```python
from build123d import *

# Parameters (mm, degrees)
F0_R      = 2.95
F1_DEPTH  = 4
F2_W      = 8.5
F2_H      = 8.5
F3_DEPTH  = 1
F4_R      = 1.5
F5_DEPTH  = 3
F7_DEPTH  = 4
F8_R      = 1.5
F9_DEPTH  = 3
F10_W     = 48
F10_H     = 4
F11_DEPTH = 1
F12_W     = 40
F12_H     = 1
F13_DEPTH = 3
F14_W     = 7
F14_H     = 7
F14_R     = 2.95
F15_DEPTH = 2


# Not quite as in the source:
# - a feature names something its author has since deleted; it is built from what else it names


with BuildPart() as f1:
    # F0 (on Top) → F1 (new body)
    with BuildSketch(Plane.XY):
        Polygon((-24, -33), (24, -33), (24, 26.5), (24, 35), (17.5, 35), (-17.5, 35), (-24, 35), (-24, 26.5), align=None)
        Circle(F0_R, mode=Mode.SUBTRACT)
    extrude(amount=F1_DEPTH)

    # F2 (on face) → F3 (cut)
    with BuildSketch(Plane(origin=(0, 0, 0), x_dir=(1, 0, 0), z_dir=(0, 0, -1))):
        with Locations((19.75, -30.75)):
            Rectangle(F2_W, F2_H)
        with Locations((-19.75, -30.75)):
            Rectangle(F2_W, F2_H)
    extrude(amount=-F3_DEPTH, mode=Mode.SUBTRACT)

    # F4 (on face) → F5 (cut)
    with BuildSketch(Plane(origin=(0, 0, 1), x_dir=(1, 0, 0), z_dir=(0, 0, -1))):
        with Locations((18.7980970389, -29.7980970389)):
            Circle(F4_R)
    extrude(amount=-F5_DEPTH, mode=Mode.SUBTRACT)

    # F6 (on face) → F7 (cut)
    with BuildSketch(Plane.XY.offset(4)):
        with BuildLine():
            Line((-18.7027541446, 3), (-11.1018016556, 3))
            ThreePointArc((-11.1018016556, 3), (-8.1134067433, 8.1500080379), (-2.95, 11.115192306))
            Line((-2.95, 11.115192306), (-2.95, 23.25))
            Line((-2.95, 23.25), (-18.7027541446, 23.25))
            Line((-18.7027541446, 23.25), (-18.7027541446, 3))
        make_face()
        with BuildLine():
            Line((2.95, 23.25), (2.95, 11.115192306))
            ThreePointArc((2.95, 11.115192306), (8.1134067433, 8.1500080379), (11.1018016556, 3))
            Line((11.1018016556, 3), (18.7027541446, 3))
            Line((18.7027541446, 3), (18.7027541446, 23.25))
            Line((18.7027541446, 23.25), (2.95, 23.25))
        make_face()
        with BuildLine():
            Line((-18.7027541446, -9.125), (-18.7027541446, -16.125))
            Line((-18.7027541446, -16.125), (-18.7027541446, -26.1487078986))
            Line((-18.7027541446, -26.1487078986), (-10, -26.1487078986))
            Line((-10, -26.1487078986), (-2.95, -26.1487078986))
            Line((-2.95, -26.1487078986), (-2.95, -11.115192306))
            ThreePointArc((-2.95, -11.115192306), (-8.1134067433, -8.1500080379), (-11.1018016556, -3))
            Line((-11.1018016556, -3), (-17.7254807204, -3))
            Line((-17.7254807204, -3), (-18.7027541446, -3))
            Line((-18.7027541446, -3), (-18.7027541446, -9.125))
        make_face()
        with BuildLine():
            ThreePointArc((11.1018016556, -3), (8.1134067433, -8.1500080379), (2.95, -11.115192306))
            Line((2.95, -11.115192306), (2.95, -26.1487078986))
            Line((2.95, -26.1487078986), (10, -26.1487078986))
            Line((10, -26.1487078986), (18.7027541446, -26.1487078986))
            Line((18.7027541446, -26.1487078986), (18.7027541446, -16.125))
            Line((18.7027541446, -16.125), (18.7027541446, -9.125))
            Line((18.7027541446, -9.125), (18.7027541446, -3.9093415253))
            Line((18.7027541446, -3.9093415253), (18.7027541446, -3))
            Line((18.7027541446, -3), (11.1018016556, -3))
        make_face()
    extrude(amount=-F7_DEPTH, mode=Mode.SUBTRACT)

    # F8 (on face) → F9 (cut)
    with BuildSketch(Plane(origin=(0, 0, 1), x_dir=(1, 0, 0), z_dir=(0, 0, -1))):
        with Locations((-18.7980970389, -29.7980970389)):
            Circle(F8_R)
    extrude(amount=-F9_DEPTH, mode=Mode.SUBTRACT)

    # F10 (on face) → F11 (cut)
    with BuildSketch(Plane(origin=(0, 0, 0), x_dir=(1, 0, 0), z_dir=(0, 0, -1))):
        with Locations((0, 31)):
            Rectangle(F10_W, F10_H)
    extrude(amount=-F11_DEPTH, mode=Mode.SUBTRACT)

    # F12 (on face) → F13 (cut)
    with BuildSketch(Plane(origin=(0, 0, 1), x_dir=(1, 0, 0), z_dir=(0, 0, -1))):
        with Locations((0, 31)):
            Rectangle(F12_W, F12_H)
    extrude(amount=-F13_DEPTH, mode=Mode.SUBTRACT)

    # F14 (on face) → F15 (cut)
    with BuildSketch(Plane.XY.offset(4)):
        Rectangle(F14_W, F14_H)
        Circle(F14_R, mode=Mode.SUBTRACT)
    extrude(amount=-F15_DEPTH, mode=Mode.SUBTRACT)


solid = f1.part
```
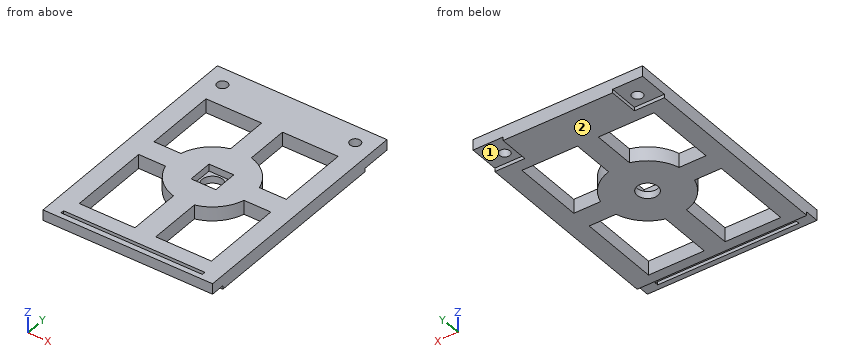
For this review, take the finished solid that the model builds, in its own axes (mm). Face numbers are marked on the shaded views. A direction names the side the tool comes from. Coordinates: 2 decimals unless noted, no trailing zeros. Loops run counter-clockwise (first coordinate to the right, second up) from the corner with the lowest first, then second, coordinate; pieces in that order, holes last.
1. Add section D-D, the plane x = 7. Give the boundary of the cut face in (y, z).
2. For line 1 (X direction, y = 18, z = 3); line 2 (Y direction, x = 0, z = 1.2); line 3 (Y direction, x = -3, z = 0.2), list the stretches that pass through material, from the lowest coordinate up.
3. Add section A-A, the plane y = -13. Give the boundary of the cut face in (x, z).
4. Add section C-C, the plane y = 0. Give the boundary of the cut face in (x, z), then the cut area to 3 significant figures.
5. Add section B-B, the plane x = 0. Give the boundary of the cut face in (y, z).
6. For the marked faces 1 and 2, list the 3-axis set-ups (+Z, -Z, +X, -X, +Y, -Y) from which the entire face can be reached by the end or side of a thin tool; tool diameter is ignored.
7. Insertion check: P1, Ø3, axis at x = 2, y = -31.5, coming from the -Z side. The pin has a flat end and moves straight along its axis. Give the tip position at first contact, or say it passes through.
Result:
1. outline: (-33, 1) - (-31.5, 1) - (-31.5, 4) - (-33, 4) - close; (-30.5, 1) - (-29, 1) - (-29, 0) - (-26.15, 0) - (-26.15, 4) - (-30.5, 4) - close; (-9.12, 0) - (9.12, 0) - (9.12, 4) - (-9.12, 4) - close; (23.25, 0) - (35, 0) - (35, 4) - (23.25, 4) - close
2. line 1: x = -24 to -18.7, -2.95 to 2.95, 18.7 to 24
2. line 2: y = -33 to -31.5, -30.5 to -2.95, 2.95 to 35
2. line 3: y = -29 to -26.15, -11.1 to 11.1, 23.25 to 35
3. outline: (-24, 0) - (-18.7, 0) - (-18.7, 4) - (-24, 4) - close; (-2.95, 0) - (2.95, 0) - (2.95, 4) - (-2.95, 4) - close; (18.7, 0) - (24, 0) - (24, 4) - (18.7, 4) - close
4. outline: (-24, 0) - (-2.95, 0) - (-2.95, 2) - (-3.5, 2) - (-3.5, 4) - (-24, 4) - close; (2.95, 0) - (24, 0) - (24, 4) - (3.5, 4) - (3.5, 2) - (2.95, 2) - close
4. area: 166 mm2
5. outline: (-33, 1) - (-31.5, 1) - (-31.5, 4) - (-33, 4) - close; (-30.5, 1) - (-29, 1) - (-29, 0) - (-2.95, 0) - (-2.95, 2) - (-3.5, 2) - (-3.5, 4) - (-30.5, 4) - close; (2.95, 0) - (35, 0) - (35, 4) - (3.5, 4) - (3.5, 2) - (2.95, 2) - close
6. face 1: -Z, +X, +Y
6. face 2: -Z, +X, -X, +Y, -Y
7. P1: stops at z = 1
